Check sheet for the modelled part. Datum: model origin and axes. Units: mm. A direction names the side the tool comes from. Coordinates: 2 decimals unless noted, no trailing zeros. Write each loop counter-clockwise with the first axis right and the second up, starting at its lowest first coordinate (ties: lowest second). Pieces come first, ordered by that corner, then holes. Notation, with made-up numbers: (75.5, -25.75) -> (109.5, -25.75) arc R34 ccw to (109.5, 8.25) -> close; hole circle Ø6 at (42, 58.25). An arc over 180 degrees is marked (long way). One line per item, written item: value. Start each with the question number.
1) Draft check along Z on faces 3 (the flat face through (32, -5.08, 25)), 4 (the cylindrical face through (29.18, -2.5, 27.04)), 5 (the cylindrical face through (34.77, 161.97, 25)), 6 (the flat face through (32, 3, 48.26)). Enter one of: +Z half, -Z half, draft (parallel to the pull), parting line (faces both ways), or undercut.
2) Sectioned sample at C-C on x = 19.5. Enter the section's corners in (y, z), plus the area to 3 significant figures.
3) Sectioned sample at B-B on x = 31.75. Enter the section's corners in (y, z).
4) Sectioned sample at D-D on z = 13.5. Enter the section's corners in (x, y), plus the area to 3 significant figures.
5) Sectioned sample at A-A on z = 25.4. Enter the section's corners in (x, y).
6) Gauge pin test, flat ends, axial feed: P1, Ø1.5, axis at x = 32, z = 31.5, coming from the -Y side; P2, Ø3.5, axis at x = 31.75, z = 25.4, coming from the +Y side. Record the tip position at first contact, or that the pin passes through.
7) Set-up check for faces 1 (the flat face through (32, 158.75, 25)), 2 (the flat face through (31, 84, 0)): record each of +Z, -Z, +X, -X, +Y, -Y from which the full face is reachable in a straight line by a thin tool's end or side.
8) Scan lines: line 1 along X through (y, z) = (162, 25); line 2 along Y through (x, z) = (46, 23.5); line 3 along Y through (x, z) = (30, 24). Record each from-to range of solid material in increasing order. Write a range as [from, to].
```python
from build123d import *

# Parameters (mm, degrees)
SKETCH1_W           = 63.5
SKETCH1_H           = 165.1
BOSS_EXTRUDE1_DEPTH = 50.8
SKETCH2_R           = 3.048
BOSS_EXTRUDE2_DEPTH = 5.08
SKETCH3_R           = 3.048
CUT_EXTRUDE1_DEPTH  = 6.35
SKETCH4_W           = 6.35
SKETCH4_H           = 6.35
CUT_EXTRUDE2_DEPTH  = 2.54


with BuildPart() as part:
    # Sketch1 → Boss-Extrude1 (new body)
    with BuildSketch(Plane.XY):
        with Locations((31.75, 82.55)):
            Rectangle(SKETCH1_W, SKETCH1_H)
    extrude(amount=BOSS_EXTRUDE1_DEPTH)

    # Sketch2 → Boss-Extrude2 (add)
    with BuildSketch(Plane.XZ):
        with Locations(Location((31.75, 25.4, 0), (0, 0, 90))):
            Circle(SKETCH2_R)
    extrude(amount=BOSS_EXTRUDE2_DEPTH)

    # Sketch3 → Cut-Extrude1 (cut)
    with BuildSketch(Plane(origin=(0, 165.1, 0), x_dir=(1, 0, 0), z_dir=(0, 1, 0))):
        with Locations(Location((31.75, -25.4, 0), (0, 0, 270))):
            Circle(SKETCH3_R)
    extrude(amount=-CUT_EXTRUDE1_DEPTH, mode=Mode.SUBTRACT)

    # Sketch4 → Cut-Extrude2 (cut)
    with BuildSketch(Plane.XY.offset(50.8)):
        with Locations((31.75, 3.175)):
            Rectangle(SKETCH4_W, SKETCH4_H)
    extrude(amount=-CUT_EXTRUDE2_DEPTH, mode=Mode.SUBTRACT)


solid = part.part
```
Answers:
1. face 3: draft
1. face 4: parting line
1. face 5: undercut
1. face 6: +Z half
2. outline: (0, 0) -> (165.1, 0) -> (165.1, 50.8) -> (0, 50.8) -> close
2. area: 8,390 mm2
3. outline: (-5.08, 22.35) -> (0, 22.35) -> (0, 0) -> (165.1, 0) -> (165.1, 22.35) -> (158.75, 22.35) -> (158.75, 28.45) -> (165.1, 28.45) -> (165.1, 50.8) -> (6.35, 50.8) -> (6.35, 48.26) -> (0, 48.26) -> (0, 28.45) -> (-5.08, 28.45) -> close
4. outline: (0, 0) -> (63.5, 0) -> (63.5, 165.1) -> (0, 165.1) -> close
4. area: 10,500 mm2
5. outline: (0, 0) -> (28.7, 0) -> (28.7, -5.08) -> (34.8, -5.08) -> (34.8, 0) -> (63.5, 0) -> (63.5, 165.1) -> (34.8, 165.1) -> (34.8, 158.75) -> (28.7, 158.75) -> (28.7, 165.1) -> (0, 165.1) -> close
6. P1: stops at y = 0
6. P2: stops at y = 158.75
7. face 1: +Y
7. face 2: -Z, +X, -X, +Y, -Y
8. line 1: x = [0, 28.73], [34.77, 63.5]
8. line 2: y = [0, 165.1]
8. line 3: y = [-5.08, 158.75]
